Geometry check sheet. Reference: the model listing, model coordinates, mm. A direction names the side the tool comes from. Give positions to 0.01 mm unless a question says otherwise; leave off trailing zeros. Order: outer loops, then holes, each group sorted by start corner. A loop starts at its lowest first (then second) coordinate and runs counter-clockwise, first axis right, second up. Notation, with made-up numbers: M 46,31 L 78,31 A14 cw 78,47 Z; hole C 3.25,68.5 d4. An arc over 180 degrees is marked long. Put each result on its own line as item: value. Start each with the question number.
Q1. Section check C-C on x = -13. Record the cut outline in (y, z), then the cut area to 3 significant figures.
Q2. Material ranges on L1, parallel to X at y = 4.4, z = 6; L2, parallel to X at y = 0.3, z = -14.5; L3, parallel to Z at x = -23, y = 4.15, recorded low to high.
Q3. Section check D-D on z = -19.5. Record the cut outline in (x, y).
Q4. Section check B-B on y = 3.1. Record the cut outline in (x, z).
Q5. Section check A-A on z = 3. Record the cut outline in (x, y).
Q6. Access from +Z, -Z, +X, -X, +Y, -Y to the whole of each face (thin tool, end or side, straight path). Record for faces 1 (the flat face through (-0.5, 3, 1)), 2 (the flat face through (-22, 3, -25)), 3 (the flat face through (-11, 3, -22)), 4 (the flat face through (-22, 3, 4)), 5 (the flat face through (0, 3, -18)).
Q7. Mould release check, pull along X, two halves, no side actions. Record for faces 6 (the flat face through (6, 3, -10)), 7 (the flat face through (-11, 3, 1)), 8 (the flat face through (-15, 3, 4)), 9 (the flat face through (-14, 0, -10)): +X half, -X half, draft (parallel to the pull), parting line (faces both ways), or undercut.
Q8. Go/stop test with flat-tipped pins: pin 1 (1.8 mm diameter, centred on y = 4.5, z = -17, fed in from +X); pin 2 (1.5 mm diameter, centred on x = -11.5, y = 2, fed in from +Z); pin 3 (3 mm diameter, centred on y = 2, z = -19.5, fed in from -X). Record where each tip stops, or that it passes through.
Autodesk Inventor part; units mm, degrees
ref_plane "YZ Plane" through (0, 0, 0) normal (1, 0, 0) x (0, 1, 0)
ref_plane "XZ Plane" through (0, 0, 0) normal (0, 1, 0) x (-1, 0, 0)
ref_plane "XY Plane" through (0, 0, 0) normal (0, 0, 1) x (1, 0, 0)
sketch "Sketch1" plane through (0, 0, 0) normal (0, 1, 0) x (-1, 0, 0)
  line L0 (0, 0) -> (35, 0)
  line L1 (35, 0) -> (35, -21)
  line L2 (35, -21) -> (0, -21)
  line L3 (0, -21) -> (0, 0)
  dimension "d0" = 35
  dimension "d1" = 21
extrude "Extrusion1" add sketch "Sketch1" along normal blind 6
sketch "Sketch2" plane through (0, 6, 0) normal (0, 1, 0) x (1, 0, 0)
  line L0 (-35, 21) -> (-35, 0)
  line L1 (-35, 0) -> (-29, 0)
  line L2 (-29, 0) -> (-29, 7)
  line L3 (-29, 7) -> (-35, 7)
  line L4 (-35, 7) -> (-35, 0)
  point P0 (0, 0)
  dimension "d4" = 6
  dimension "d5" = 7
extrude "Extrusion2" cut sketch "Sketch2" against normal blind 6
pattern_linear "Rectangular Pattern1" count 2 spacing 14 along (0, 0, -1) of "Extrusion2"
sketch "Sketch3" plane through (0, 6, 0) normal (0, 1, 0) x (1, 0, 0)
  line L0 (-29, 7) -> (-29, 0)
  line L1 (-29, 0) -> (0, 0)
  line L2 (0, 0) -> (0, -1)
  line L3 (0, -1) -> (-29, -1)
  line L4 (-29, -1) -> (-29, 0)
  line L5 (-29, 14) -> (-29, 21)
  line L6 (-29, 21) -> (0, 21)
  line L7 (0, 21) -> (0, 22)
  line L8 (0, 22) -> (-29, 22)
  line L9 (-29, 22) -> (-29, 21)
  point P0 (0, 0)
  dimension "d11" = 29
  dimension "d12" = 1
  dimension "d13" = 29
  dimension "d14" = 1
extrude "Extrusion3" add sketch "Sketch3" against normal blind 6
sketch "Sketch4" plane through (0, 6, 0) normal (0, 1, 0) x (1, 0, 0)
  line L0 (-29, -1) -> (-29, 7)
  line L1 (0, 22) -> (0, -1)
  line L2 (0, 7) -> (6, 7)
  line L3 (6, 7) -> (6, 14)
  line L4 (6, 14) -> (0, 14)
  line L5 (0, 14) -> (0, 7)
  point P0 (0, 0)
  dimension "d17" = 6
  dimension "d18" = 7
extrude "Extrusion4" add sketch "Sketch4" against normal blind 6
sketch "Sketch5" plane through (0, 6, 0) normal (0, 1, 0) x (1, 0, 0)
  line L0 (0, -1) -> (-29, -1)
  line L1 (-29, -1) -> (-22, -1)
  line L2 (-22, -1) -> (-22, -7)
  line L3 (-22, -7) -> (-15, -7)
  line L4 (-15, -7) -> (-15, -1)
  line L5 (-29, 22) -> (0, 22)
  line L6 (-29, 22) -> (-22, 22)
  line L7 (-22, 22) -> (-22, 28)
  line L8 (-22, 28) -> (-15, 28)
  line L9 (-15, 28) -> (-15, 22)
  point P0 (0, 0)
  dimension "d22" = 6
  dimension "d23" = 7
  dimension "d25" = 6
  dimension "d26" = 7
extrude "Extrusion5" add sketch "Sketch5" against normal blind 6
pattern_linear "Rectangular Pattern2" count 2 spacing 14 along (1, 0, 0) of "Extrusion5"
properties part number "g_arm 2"
Results found:
1. outline: M 0,-22 L 6,-22 L 6,1 L 0,1 Z
1. area: 138 mm^2
2. L1: x = -22 to -15, -8 to -1
2. L2: x = -29 to 0
2. L3: z = -22 to 1
3. outline: M -29,0 L 0,0 L 0,6 L -29,6 Z
4. outline: M -35,-14 L -29,-14 L -29,-22 L -22,-22 L -22,-28 L -15,-28 L -15,-22 L -8,-22 L -8,-28 L -1,-28 L -1,-22 L 0,-22 L 0,-14 L 6,-14 L 6,-7 L 0,-7 L 0,1 L -1,1 L -1,7 L -8,7 L -8,1 L -15,1 L -15,7 L -22,7 L -22,1 L -29,1 L -29,-7 L -35,-7 Z
5. outline: M -22,0 L -15,0 L -15,6 L -22,6 Z; M -8,0 L -1,0 L -1,6 L -8,6 Z
6. face 1: +Z, +X, +Y, -Y
6. face 2: -Z, -X, +Y, -Y
6. face 3: -Z, +Y, -Y
6. face 4: +Z, -X, +Y, -Y
6. face 5: -Z, +X, +Y, -Y
7. face 6: +X half
7. face 7: undercut
7. face 8: undercut
7. face 9: draft
8. pin 1: stops at x = 0
8. pin 2: stops at z = 1
8. pin 3: stops at x = -29
